Work out the finished part from the listing and answer in its coordinate system (mm). A direction names the side the tool comes from. Coordinates: 2 decimals unless noted, no trailing zeros. Write each loop counter-clockwise with the first axis right and the second up, starting at its lowest first coordinate (ties: lowest second). Pieces come first, ordered by that corner, then holes. Notation, with made-up numbers: (31.5, 17) - (39.5, 17) arc R31 ccw to (39.5, 52) - close; hole circle Ø4 at (-12.5, 5.25). An arc over 180 degrees is marked (long way). One line per item, written item: value.
```python
from build123d import *

# Parameters (mm, degrees)
BOSS_EXTRUDE1_DEPTH = 10
BOSS_EXTRUDE2_DEPTH = 5


with BuildPart() as part:
    # Sketch2 → Boss-Extrude1 (new body)
    with BuildSketch(Plane.XY):
        Polygon((77.769059892, 108.719200877), (133.038119785, 12.990381057), (125.769059892, 0.4), (15.230940108, 0.4), (13.562177826, 3.290381057), (14.780166891, 5.4), (122.882308546, 5.4), (127.264617093, 12.990381057), (73.213546265, 106.609581934), (74.43153533, 108.719200877), align=None)
    extrude(amount=-BOSS_EXTRUDE1_DEPTH)

    # Sketch3 → Boss-Extrude2 (add)
    with BuildSketch(Plane.XY):
        Polygon((58.381197846, 114.119200877), (82.618802154, 114.119200877), (142.504165125, 10.394709581), (132.75, -6.5), (12.979274058, -6.5), (0.860471904, 14.490381057), align=None)
    extrude(amount=BOSS_EXTRUDE2_DEPTH)


solid = part.part
```
Item 1: Section A-A, the plane z = -4 is taken. Determine the outline of the cut face in (x, y), then the cut area to 3 significant figures.
Evaluation:
outline: (13.56, 3.29) - (15.23, 0.4) - (125.77, 0.4) - (133.04, 12.99) - (77.77, 108.72) - (74.43, 108.72) - (73.21, 106.61) - (127.26, 12.99) - (122.88, 5.4) - (14.78, 5.4) - close
area: 1,160 mm2
Item 2: Section D-D, the plane z = 3.5 is taken. Determine the outline of the cut face in (x, y), then the cut area to 3 significant figures.
Evaluation:
outline: (0.86, 14.49) - (12.98, -6.5) - (132.75, -6.5) - (142.5, 10.39) - (82.62, 114.12) - (58.38, 114.12) - close
area: 10,900 mm2
Item 3: Which of the six approach directions +Z, -Z, +X, -X, +Y, -Y give full straight-line access (tool end or side, diameter ignored) to faces 1 (the face through (14.41, 1.82, -4.93)), 2 (the face through (100.62, 59.14, -4.93)), 3 (the face through (71, 0.4, -5)), 4 (the face through (76, 108.719, -5))?
Evaluation:
face 1: -Z, -X, -Y
face 2: -Z, -X
face 3: -Z, +X, -X, -Y
face 4: -Z, +X, -X, +Y
Item 4: Section C-C, the plane x = 42 is taken. Determine the outline of the cut face in (y, z).
Evaluation:
outline: (-6.5, 0) - (0.4, 0) - (0.4, -10) - (5.4, -10) - (5.4, 0) - (85.75, 0) - (85.75, 5) - (-6.5, 5) - close
Item 5: Section B-B, the plane y = 57 is taken. Determine the outline of the cut face in (x, z).
Evaluation:
outline: (25.4, 0) - (101.86, 0) - (101.86, -10) - (107.63, -10) - (107.63, 0) - (115.6, 0) - (115.6, 5) - (25.4, 5) - close
Item 6: Determine the mould class of faces 5 (the face through (105.02, 61.52, -4.93)), 6 (the face through (137.7, 2.07, 2.46)), 7 (the face through (73, 41, 0)) for opening direction Y: +Y half, -Y half, draft (parallel to the pull), parting line (faces both ways), or undercut.
Evaluation:
face 5: +Y half
face 6: -Y half
face 7: undercut
Item 7: Consider probe 1 along Y at (x, z) = (26, -4); probe 2 along Z at (x, y) = (108, 44.5); probe 3 along Y at (x, z) = (87, -8.5). Determine where each line is inside the solid, lowest interval first.
Evaluation:
probe 1: y = 0.4 to 5.4
probe 2: z = 0 to 5
probe 3: y = 0.4 to 5.4, 82.73 to 92.73
Item 8: Given pin 1 (5 mm diameter, centred on y = 82, z = -3.5, fed in from +X); pin 2 (3 mm diameter, centred on y = 72, z = -6.5, fed in from +X); pin 3 (8 mm diameter, centred on x = 81.5, y = 68.5, fed in from -Z), each flat-ended and moving along its own axis, determine where each tip first touches the part or whether it passes through.
Evaluation:
pin 1: stops at x = 94.64
pin 2: stops at x = 99.83
pin 3: stops at z = 0
